Input: dimensioned drawing with shaded views. Units: mm. Origin: part minimum x, y, z. A direction names the side the tool comes from. Coordinates: 2 decimals unless noted, no trailing zeros. Order: outer loops, then holes, each group sorted by start corner. A loop starts at its lowest first (then second) coordinate and runs counter-clockwise, first axis right, second up.
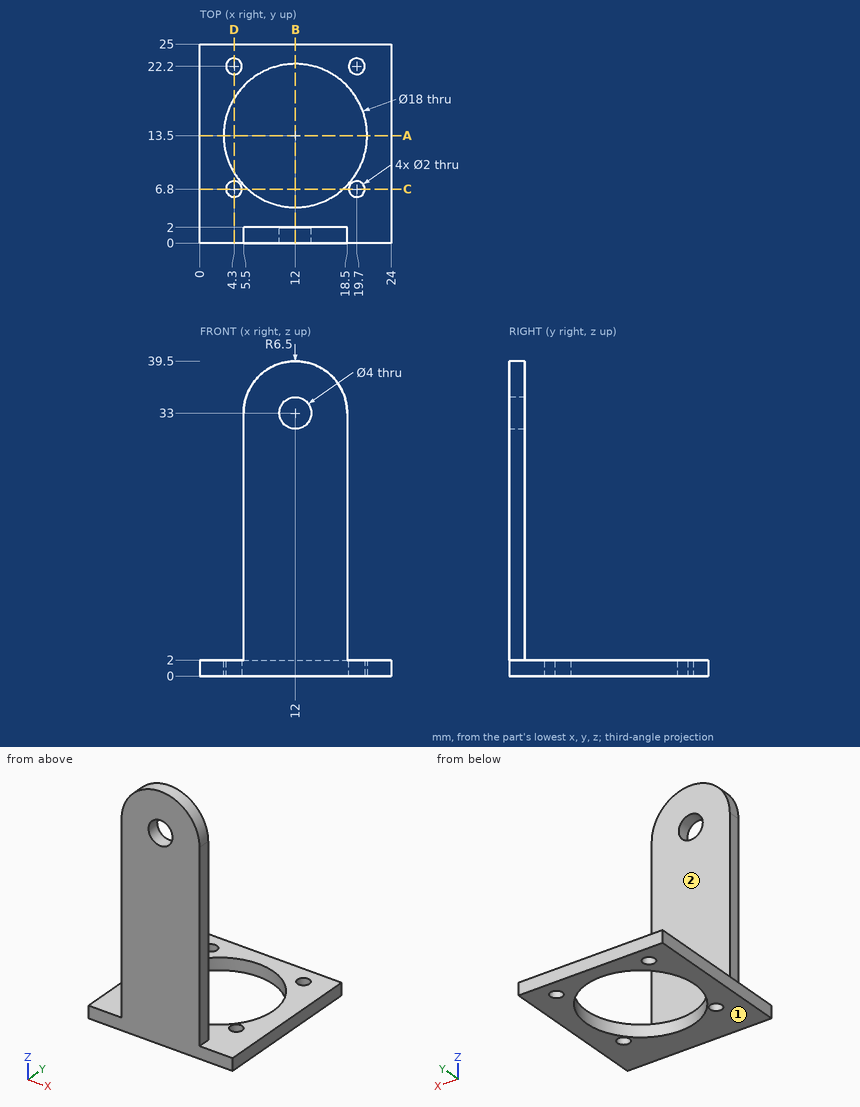
1. Section query D-D, the plane x = 4.3. Output: boundary loops of the cut face in (y, z), plus the area to 3 significant figures.
2. Section query B-B, the plane x = 12. Output: boundary loops of the cut face in (y, z), plus the area to 3 significant figures.
3. Material intervals for line 1 along Y through (x, z) = (12, 1.2); line 2 along X through (y, z) = (0.85, 33); line 3 along Y through (x, z) = (6.5, 13), sorted ascending.
4. Access query for the marked faces 1 and 2. Directions: +Z, -Z, +X, -X, +Y, -Y. A direction counts if a zero-diameter tool reaches every point of the face in a straight line with its end or side. Return the directions, or none.
5. Section query A-A, the plane y = 13.5. Output: boundary loops of the cut face in (x, z), plus the area to 3 significant figures.
6. Section query C-C, the plane y = 6.8. Output: boundary loops of the cut face in (x, z), plus the area to 3 significant figures.
7. Contact query for flat-ended pins moving along their axis: P1, Ø2, axis at x = 21, y = 14, coming from the +Z side; P2, Ø3, axis at x = 18.5, z = 24.5, coming from the +Y side; P3, Ø1.8, axis at x = 4.3, y = 22.2, coming from the +Z side; P4, Ø1, axis at y = 1, z = 13, coming from the -X side. Output: stop coordinate, or through.
Answer key:
1. outline: (0, 0) - (5.8, 0) - (5.8, 2) - (0, 2) - close; (7.8, 0) - (8.84, 0) - (8.84, 2) - (7.8, 2) - close; (18.16, 0) - (21.2, 0) - (21.2, 2) - (18.16, 2) - close; (23.2, 0) - (25, 0) - (25, 2) - (23.2, 2) - close
1. area: 23.4 mm2
2. outline: (0, 0) - (4.5, 0) - (4.5, 2) - (2, 2) - (2, 31) - (0, 31) - close; (0, 35) - (2, 35) - (2, 39.5) - (0, 39.5) - close; (22.5, 0) - (25, 0) - (25, 2) - (22.5, 2) - close
2. area: 81.0 mm2
3. line 1: y = 0 to 4.5, 22.5 to 25
3. line 2: x = 5.5 to 10, 14 to 18.5
3. line 3: y = 0 to 2
4. face 1: -Z, +X, -X, +Y, -Y
4. face 2: +Z, +X, -X, +Y
5. outline: (0, 0) - (3, 0) - (3, 2) - (0, 2) - close; (21, 0) - (24, 0) - (24, 2) - (21, 2) - close
5. area: 12.0 mm2
6. outline: (0, 0) - (3.3, 0) - (3.3, 2) - (0, 2) - close; (5.3, 0) - (5.99, 0) - (5.99, 2) - (5.3, 2) - close; (18.01, 0) - (18.7, 0) - (18.7, 2) - (18.01, 2) - close; (20.7, 0) - (24, 0) - (24, 2) - (20.7, 2) - close
6. area: 16.0 mm2
7. P1: stops at z = 2
7. P2: stops at y = 2
7. P3: passes through
7. P4: stops at x = 5.5
